Read the model definition and answer for the solid it produces. Units are mm, in the model's axes. A direction names the side the tool comes from. Round coordinates to 2 decimals unless told otherwise and drop trailing zeros. Order: outer loops, then holes, each group sorted by start corner. A loop starts at its lowest first (then second) coordinate and runs counter-clockwise, first axis right, second up.
from build123d import *

# Parameters (mm, degrees)
SKETCH2_W           = 100
SKETCH2_H           = 15
BOSS_EXTRUDE1_DEPTH = 3.25
SKETCH4_R           = 1.45
BOSS_EXTRUDE2_DEPTH = 4
SKETCH5_R           = 5.1
CUT_EXTRUDE1_DEPTH  = 4
FILLET1_R           = 1
SKETCH6_W           = 8.5
SKETCH6_H           = 4
SKETCH6_W_2         = 5
SKETCH6_H_2         = 3.25
CUT_EXTRUDE3_DEPTH  = 1.125


with BuildPart() as part:
    # Sketch2 → Boss-Extrude1 (new, symmetric)
    with BuildSketch(Plane(origin=(0, 0, 0), x_dir=(1, 0, 0), z_dir=(0, 1, 0))):
        Rectangle(SKETCH2_W, SKETCH2_H)
    extrude(amount=BOSS_EXTRUDE1_DEPTH, both=True)

    # Sketch4 → Boss-Extrude2 (add)
    with BuildSketch(Plane(origin=(0, 3.25, 0), x_dir=(1, 0, 0), z_dir=(0, 1, 0))):
        with Locations(Location((45, 0, 0), (0, 0, 90))):
            Circle(SKETCH4_R)
    extrude(amount=BOSS_EXTRUDE2_DEPTH)

    # Sketch5 → Cut-Extrude1 (cut)
    with BuildSketch(Plane(origin=(0, -3.25, 0), x_dir=(-1, 0, 0), z_dir=(0, -1, 0))):
        with Locations(Location((40, 0, 0), (0, 0, 90))):
            Circle(SKETCH5_R)
    extrude(amount=-CUT_EXTRUDE1_DEPTH, mode=Mode.SUBTRACT)

    # Fillet1
    fillet1_edges = [part.edges().sort_by_distance(p)[0] for p in [
        (45, 3.25, 1.45),
    ]]
    fillet(fillet1_edges, radius=FILLET1_R)

    # Sketch6 → Cut-Extrude3 (cut, symmetric)
    with BuildSketch(Plane.XY):
        with Locations((-19.25, -1.25)):
            Rectangle(SKETCH6_W, SKETCH6_H)
        with Locations((-12.5, -0.875)):
            Rectangle(SKETCH6_W_2, SKETCH6_H_2)
    extrude(amount=CUT_EXTRUDE3_DEPTH, both=True, mode=Mode.SUBTRACT)


solid = part.part
Q1. Straight lines are drawn through the part: probe 1 along X at (y, z) = (-0.4, 0); probe 2 along Z at (x, y) = (-23, -1) (3 decimals); probe 3 along Z at (x, y) = (45, 4.25). For each, find the intervals that lie inside material, in ascending order.
Outcome:
probe 1: x = -50 to -45.1, -34.9 to -23.5, -10 to 50
probe 2: z = -7.5 to -1.125, 1.125 to 7.5
probe 3: z = -1.45 to 1.45
Q2. For faces 4 (the face through (-38.468, -1.278, -4.864)), 5 (the face through (-17, -1, 1.125)), 6 (the face through (-1, -3.25, 0)), determine the directions among +Z, -Z, +X, -X, +Y, -Y from which every point of the face is accessible in a straight line to the end or side of a thin tool.
Outcome:
face 4: -Y
face 5: none
face 6: +Z, -Z, +X, -X, -Y
Q3. A cutting plane is placed at C-C, the plane y = 5.5. Give the vertices of the cut face in (x, z).
Outcome:
outline: circle Ø2.9 at (45, 0)
Q4. For a pull along Z with two mould halves and no side action, classify faces 1 (the face through (-23.5, -1, 0)), 2 (the face through (46.286, 5.729, -0.669)), 3 (the face through (-1, 0, -7.5)) as released by +Z, released by -Z, zero draft, split by the parting line, or undercut.
Outcome:
face 1: undercut
face 2: split by the parting line
face 3: released by -Z
Q5. A cutting plane is placed at B-B, the plane z = 0. Give the vertices of the cut face in (x, y).
Outcome:
outline: (-50, -3.25) - (-45.1, -3.25) - (-45.1, 0.75) - (-34.9, 0.75) - (-34.9, -3.25) - (-23.5, -3.25) - (-23.5, 0.75) - (-10, 0.75) - (-10, -2.5) - (-15, -2.5) - (-15, -3.25) - (50, -3.25) - (50, 3.25) - (47.45, 3.25) arc R1 cw to (46.45, 4.25) - (46.45, 7.25) - (43.55, 7.25) - (43.55, 4.25) arc R1 cw to (42.55, 3.25) - (-50, 3.25) - close
Q6. A cutting plane is placed at A-A, the plane x = -40. Give the vertices of the cut face in (y, z), plus the area to 3 significant figures.
Outcome:
outline: (-3.25, -7.5) - (3.25, -7.5) - (3.25, 7.5) - (-3.25, 7.5) - (-3.25, 5.1) - (0.75, 5.1) - (0.75, -5.1) - (-3.25, -5.1) - close
area: 56.7 mm2
Q7. A cutting plane is placed at D-D, the plane x = 45. Give the vertices of the cut face in (y, z).
Outcome:
outline: (-3.25, -7.5) - (3.25, -7.5) - (3.25, -2.45) arc R1 cw to (4.25, -1.45) - (7.25, -1.45) - (7.25, 1.45) - (4.25, 1.45) arc R1 cw to (3.25, 2.45) - (3.25, 7.5) - (-3.25, 7.5) - close
Q8. Flat-ended cylindrical pins translate along their axes: pin 1 (0.7 mm diameter, centred on x = -12, z = 0, fed in from +Y); pin 2 (3 mm diameter, centred on x = -38, z = 0.5, fed in from -Y). Find the tip coordinate at first contact, or state that the pin passes through.
Outcome:
pin 1: stops at y = 3.25
pin 2: stops at y = 0.75
